```python
from build123d import *

# Parameters (mm, degrees)
BOSS_EXTRUDE1_DEPTH = 1.875
BOSS_EXTRUDE2_DEPTH = 11.25
SKETCH4_R           = 10
CUT_EXTRUDE1_DEPTH  = 28.230497608
THREAD1_PITCH       = 4


with BuildPart() as part:
    # Sketch1 → Boss-Extrude1 (new, symmetric)
    with BuildSketch(Plane(origin=(0, 0, 0), x_dir=(1, 0, 0), z_dir=(0, 1, 0))):
        with BuildLine():
            Line((-14.5, 9.797958971), (-14.5, -9.797958971))
            ThreePointArc((-14.5, -9.797958971), (0, -17.5), (14.5, -9.797958971))
            Line((14.5, -9.797958971), (14.5, 9.797958971))
            ThreePointArc((14.5, 9.797958971), (0, 17.5), (-14.5, 9.797958971))
        make_face()
    extrude(amount=BOSS_EXTRUDE1_DEPTH, both=True)

    # Sketch2 → Boss-Extrude2 (add)
    with BuildSketch(Plane(origin=(0, 1.875, 0), x_dir=(1, 0, 0), z_dir=(0, 1, 0))):
        with BuildLine():
            Line((12, 9), (12, -9))
            ThreePointArc((12, -9), (0, -15), (-12, -9))
            Line((-12, -9), (-12, 9))
            ThreePointArc((-12, 9), (0, 15), (12, 9))
        make_face()
    extrude(amount=BOSS_EXTRUDE2_DEPTH)

    # Sketch4 → Cut-Extrude1 (cut, through all)
    with BuildSketch(Plane(origin=(0, 13.125, 0), x_dir=(1, 0, 0), z_dir=(0, 1, 0))):
        with Locations(Location((0, 0, 0), (0, 0, 270))):
            Circle(SKETCH4_R)
    extrude(amount=-CUT_EXTRUDE1_DEPTH, mode=Mode.SUBTRACT)

    # Thread1: arcs per turn and ends read off the stored shape
    # Thread1: the profile of Thread Profile1 profile screwed along a right-hand helix through 3 turns, 12 arcs to a turn; built about Z, then put on its axis
    thread1_z = Axis((0, 0, 0), (0, 0, 1))
    thread1_corners = [(10.0003, 0, -0.000173205), (7.8349365, 0, 1.249999995), (7.8349365, 0, 1.749999995), (10.0003, 0, 3.000173194)]
    with BuildLine(mode=Mode.PRIVATE) as thread1_profile:
        Line(thread1_corners[0], thread1_corners[1])
        Line(thread1_corners[1], thread1_corners[2])
        Line(thread1_corners[2], thread1_corners[3])
        Line(thread1_corners[3], thread1_corners[0])
    thread1_cap = Face(thread1_profile.wire())
    thread1_turn_angles = [0, 15, 30, 45, 60, 75, 90, 105, 120, 135, 150, 165, 180, 195, 210, 225, 240, 255, 270, 285, 300, 315, 330, 345, 360]
    thread1_turn_weights = [1, 0.9659258262890683, 1, 0.9659258262890683, 1, 0.9659258262890683, 1, 0.9659258262890683, 1, 0.9659258262890683, 1, 0.9659258262890683, 1, 0.9659258262890683, 1, 0.9659258262890683, 1, 0.9659258262890683, 1, 0.9659258262890683, 1, 0.9659258262890683, 1, 0.9659258262890683, 1]
    thread1_turn_rails = [Edge.make_bspline([Vector(p[0], p[1], 0).rotate(thread1_z, thread1_turn_angles[k]) / thread1_turn_weights[k] + Vector(0, 0, p[2] + THREAD1_PITCH * thread1_turn_angles[k] / 360) for k in range(25)], [0, 0, 0, 1, 1, 2, 2, 3, 3, 4, 4, 5, 5, 6, 6, 7, 7, 8, 8, 9, 9, 10, 10, 11, 11, 12, 12, 12], 2, thread1_turn_weights) for p in thread1_corners]
    thread1_turn_sides = [Face.make_surface_from_curves(thread1_turn_rails[p[0]], thread1_turn_rails[p[1]]) for p in [(0, 1), (1, 2), (2, 3), (3, 0)]]
    thread1 = Plane(origin=(0, 13.125, 0), x_dir=(-1, 0, 0), z_dir=(0, -1, 0)) * Solid(Shell([*[p.moved(Location((0, 0, THREAD1_PITCH * i))) for i in range(3) for p in thread1_turn_sides], thread1_cap, thread1_cap.rotate(thread1_z, 1080).moved(Location((0, 0, THREAD1_PITCH * 1080 / 360)))]))
    add(thread1)


solid = part.part
```
Here's how the part is built. I have some questions about the finished solid (model axes, mm). A direction names the side the tool comes from. Round coordinates to 2 decimals unless told otherwise and drop trailing zeros. Loops run counter-clockwise (first coordinate to the right, second up) from the corner with the lowest first, then second, coordinate; pieces in that order, holes last.
1. Suppose I cut it at C-C, the plane x = 9.5. Give the number of separate pieces and of enclosed holes in the cut face, and give its area (3 significant figures).
Answers:
separate pieces: 1
enclosed holes: 2
area: 327 mm2
2. Thinking about a two-plate mould opening in Z: for faces 1 (the face through (-9, 0, 0)), 2 (the face through (-0.2, 0, 17.5)), 3 (the face through (0, 7, -15)), which applies, released by +Z, released by -Z, zero draft, split by the parting line, or undercut?
Answers:
face 1: undercut
face 2: released by +Z
face 3: released by -Z
3. For faces 4 (the face through (-13, 1.875, 1)), 5 (the face through (12, 7, 0)), 6 (the face through (-12, 7, 0)), 7 (the face through (0, 7, 15)), which set-ups out of +Z, -Z, +X, -X, +Y, -Y let a thin tool reach every point of the face, with its end or its side?
Answers:
face 4: +Y
face 5: +Z, -Z, +X, +Y
face 6: +Z, -Z, -X, +Y
face 7: +Z, +Y
4. Suppose I cut it at A-A, the plane z = -13.5. Please give me the cut outline in (x, y) (3 decimals), and give its area (3 significant figures).
Answers:
outline: (-11.136, -1.875) - (11.136, -1.875) - (11.136, 1.875) - (6.538, 1.875) - (6.538, 13.125) - (-6.538, 13.125) - (-6.538, 1.875) - (-11.136, 1.875) - close
area: 231 mm2
5. Suppose I cut it at B-B, the plane x = -11. Please give me the cut outline in (y, z) (3 decimals), and give its area (3 significant figures).
Answers:
outline: (-1.875, -13.611) - (1.875, -13.611) - (1.875, -10.198) - (13.125, -10.198) - (13.125, 10.198) - (1.875, 10.198) - (1.875, 13.611) - (-1.875, 13.611) - close
area: 332 mm2
6. If I drill on probe 1 along Y at (x, z) = (7.25, -6.5); probe 2 along Y at (x, z) = (-2, -16) (3 decimals); probe 3 along Z at (x, y) = (3.5, 12.75), over which ranges is the centre line in solid material (lowest first)?
Answers:
probe 1: y = 0.74 to 3.44, 4.74 to 7.44, 8.74 to 11.44
probe 2: y = -1.875 to 1.875
probe 3: z = -14.59 to -9.37, 9.37 to 14.59
7. Will these pins go through, and if not, where does the flat tip stop? pin 1 (3 mm diameter, centred on x = 8.5, y = 4.5, fed in from -Z); pin 2 (2 mm diameter, centred on y = 9, z = -4.5, fed in from +X); pin 3 (1.7 mm diameter, centred on x = -9, y = 0, fed in from -Z).
Answers:
pin 1: stops at z = -13.27
pin 2: stops at x = 12
pin 3: stops at z = -15.49
